from build123d import *

# Parameters (mm, degrees)
SKETCH1_W           = 95
SKETCH1_H           = 60
BOSS_EXTRUDE1_DEPTH = 0.5
SKETCH2_W           = 95
SKETCH2_H           = 60
SKETCH2_W_2         = 94
SKETCH2_H_2         = 59
BOSS_EXTRUDE2_DEPTH = 10.5
SKETCH3_W           = 97.06
SKETCH3_H           = 62.06
SKETCH3_W_2         = 94
SKETCH3_H_2         = 59
BOSS_EXTRUDE3_DEPTH = 1.5
FILLET2_R           = 12
FILLET3_R           = 12
FILLET4_R           = 0.749
SKETCH4_W           = 12.1
SKETCH4_H           = 1.5
CUT_EXTRUDE1_DEPTH  = 0.5


with BuildPart() as part:
    # Sketch1 → Boss-Extrude1 (new body)
    with BuildSketch(Plane(origin=(0, 0, 0), x_dir=(1, 0, 0), z_dir=(0, 1, 0))):
        Rectangle(SKETCH1_W, SKETCH1_H)
    extrude(amount=BOSS_EXTRUDE1_DEPTH)

    # Sketch2 → Boss-Extrude2 (add)
    with BuildSketch(Plane(origin=(0, 0.5, 0), x_dir=(1, 0, 0), z_dir=(0, 1, 0))):
        Rectangle(SKETCH2_W, SKETCH2_H)
        Rectangle(SKETCH2_W_2, SKETCH2_H_2, mode=Mode.SUBTRACT)
    extrude(amount=BOSS_EXTRUDE2_DEPTH)

    # Sketch3 → Boss-Extrude3 (add)
    with BuildSketch(Plane(origin=(0, 11, 0), x_dir=(1, 0, 0), z_dir=(0, 1, 0))):
        Rectangle(SKETCH3_W, SKETCH3_H)
        Rectangle(SKETCH3_W_2, SKETCH3_H_2, mode=Mode.SUBTRACT)
    extrude(amount=BOSS_EXTRUDE3_DEPTH)

    # Fillet2
    fillet2_edges = [part.edges().sort_by_distance(p)[0] for p in [
        (-47, 6.5, 29.5),
        (47, 6.5, -29.5),
        (47, 6.5, 29.5),
        (-47.5, 5.5, -30),
    ]]
    fillet(fillet2_edges, radius=FILLET2_R)

    # Fillet3
    fillet3_edges = [part.edges().sort_by_distance(p)[0] for p in [
        (-47, 6.5, -29.5),
        (-48.53, 11.75, -31.03),
        (-48.53, 11.75, 31.03),
        (48.53, 11.75, 31.03),
        (48.53, 11.75, -31.03),
        (47.5, 5.5, -30),
        (47.5, 5.5, 30),
        (-47.5, 5.5, 30),
    ]]
    fillet(fillet3_edges, radius=FILLET3_R)

    # Fillet4
    fillet4_edges = [part.edges().sort_by_distance(p)[0] for p in [
        (0, 11, 31.03),
        (0, 12.5, 31.03),
        (-48.53, 11, 0),
        (-48.53, 12.5, 0),
        (48.53, 12.5, 0),
        (0, 12.5, -31.03),
        (-47, 12.5, 0),
        (45.015281374, 12.5, 27.515281374),
        (45.015281374, 12.5, -27.515281374),
        (-45.015281374, 12.5, 27.515281374),
        (0, 11, -31.03),
        (48.53, 11, 0),
        (-45.015281374, 11, -27.515281374),
        (-43.485281374, 12.5, -25.985281374),
        (45.015281374, 11, 27.515281374),
        (45.015281374, 11, -27.515281374),
        (-45.015281374, 11, 27.515281374),
        (-45.015281374, 12.5, -27.515281374),
        (47, 12.5, 0),
        (0, 12.5, -29.5),
        (0, 12.5, 29.5),
        (43.485281374, 12.5, -25.985281374),
        (43.485281374, 12.5, 25.985281374),
        (-43.485281374, 12.5, 25.985281374),
    ]]
    fillet(fillet4_edges, radius=FILLET4_R)

    # Sketch4 → Cut-Extrude1 (cut)
    with BuildSketch(Plane(origin=(0, 0, 29.5), x_dir=(-1, 0, 0), z_dir=(0, 0, -1))):
        with Locations((-21.45, 9.75)):
            Rectangle(SKETCH4_W, SKETCH4_H)
        with Locations((21.45, 9.75)):
            Rectangle(SKETCH4_W, SKETCH4_H)
    extrude(amount=-CUT_EXTRUDE1_DEPTH, mode=Mode.SUBTRACT)


solid = part.part
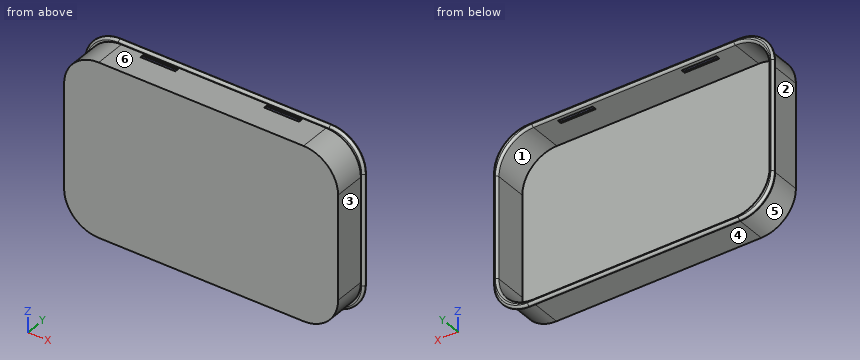
Check sheet for the modelled part. Datum: model origin and axes. Units: mm. Face numbers are marked on the shaded views. A direction names the side the tool comes from. Give positions to 0.01 mm unless a question says otherwise; leave off trailing zeros. Loops run counter-clockwise (first coordinate to the right, second up) from the corner with the lowest first, then second, coordinate; pieces in that order, holes last. Notation, with made-up numbers: M 34.25,54 L 47.25,54 A12 cw 47.25,60 Z; hole C 4,38.25 d11. An arc over 180 degrees is marked long. Use a Markdown table: item, result. Add a question column.
Q1. Tool access check on the marked faces 4, 5 and 6. Record the directions out of +Z, -Z, +X, -X, +Y, -Y that give a thin tool (end or side, any length) a straight path to the whole face; none if there is none.
Q2. Mould release check, pull along X, two halves, no side actions. Record for the marked faces 1, 2 and 3: pulls with the +X half, pulls with the -X half, needs draft (parallel to the pull), parting line crosses it, or undercut.
Q3. Scan lines: line 1 along Z through (x, y) = (4, 7.5); line 2 along X through (y, z) = (2.25, -10); line 3 along Y through (x, z) = (-21, -5). Record each from-to range of solid material in increasing order. Write a range as [from, to].
Q4. Go/stop test with flat-tipped pins: pin 1 (3.5 mm diameter, centred on y = 4, z = 5.5, fed in from +X); pin 2 (5.5 mm diameter, centred on x = -7.5, y = 4.5, fed in from +Z); pin 3 (5 mm diameter, centred on y = 4, z = 0.5, fed in from -X). Record where each tip stops, or that it passes through.
Q5. Sectioned sample at B-B, the plane y = 3.75. Record the cut outline in (x, z), then the cut area to 3 significant figures.
Verdict:
| question | item | result |
|---|---|---|
| 1 | face 4 | -Z, +X, -X, -Y |
| 1 | face 5 | -Z, -X, -Y |
| 1 | face 6 | +Z, +X, -X, -Y |
| 2 | face 1 | undercut |
| 2 | face 2 | pulls with the -X half |
| 2 | face 3 | pulls with the +X half |
| 3 | line 1 | [-30, -29.5], [29.5, 30] |
| 3 | line 2 | [-47.5, -47], [47, 47.5] |
| 3 | line 3 | [0, 0.5] |
| 4 | pin 1 | x = 47.5 |
| 4 | pin 2 | z = 30 |
| 4 | pin 3 | x = -47.5 |
| 5 | outline | M -47.5,-18 A12 ccw -35.5,-30 L 35.5,-30 A12 ccw 47.5,-18 L 47.5,18 A12 ccw 35.5,30 L -35.5,30 A12 ccw -47.5,18 Z; hole M -47,-17.5 A12 ccw -35,-29.5 L 35,-29.5 A12 ccw 47,-17.5 L 47,17.5 A12 ccw 35,29.5 L -35,29.5 A12 ccw -47,17.5 Z |
| 5 | area | 154 mm^2 |
